Autodesk Inventor part; units mm, degrees
ref_plane "YZ Plane" through (0, 0, 0) normal (1, 0, 0) x (0, 1, 0)
ref_plane "XZ Plane" through (0, 0, 0) normal (0, 1, 0) x (-1, 0, 0)
ref_plane "XY Plane" through (0, 0, 0) normal (0, 0, 1) x (1, 0, 0)
sketch "Sketch1" plane through (0, 0, 0) normal (1, 0, 0) x (0, 1, 0)
  line L0 (0, 0) -> (12.4509, 21.5656)
  line L1 (12.4509, 21.5656) -> (46.5463, 1.8806)
  line L2 (0, -101.8491) -> (0, 42.1347)
  line L3 (46.5463, 1.8806) -> (0, -78.74)
  line L4 (0, 0) -> (0, -78.74)
  line L5 (19.05, 17.7556) -> (0, -15.24) construction
  dimension "d0" = 39.37
  dimension "d1" = 30
  dimension "d5" = 7.62
  dimension "d6" = 38.1
extrude "Extrusion1" add sketch "Sketch1" along normal mid plane 39.37
sketch "Sketch2" plane through (-19.685, 12.4509, 21.5656) normal (0, 0.5, 0.866) x (1, 0, 0)
  line L0 (0, 0) -> (39.37, 0) construction
  line L1 (39.37, 0) -> (39.37, 39.37) construction
  line L2 (0, 0) -> (39.37, 39.37) construction
  line L3 (39.37, 39.37) -> (0, 39.37) construction
  line L4 (0, 39.37) -> (39.37, 0) construction
  line L5 (6.35, 6.35) -> (33.02, 6.35)
  line L6 (33.02, 6.35) -> (33.02, 33.02)
  line L7 (33.02, 33.02) -> (6.35, 33.02)
  line L8 (6.35, 33.02) -> (6.35, 6.35)
  line L9 (6.35, 6.35) -> (33.02, 33.02) construction
  line L10 (33.02, 6.35) -> (6.35, 33.02) construction
  point P0 (19.685, 0)
  point P1 (19.685, 19.685)
  dimension "d7" = 26.67
extrude "Extrusion2" cut sketch "Sketch2" against normal blind 38.1
sketch "Sketch3" plane through (0, 0, 0) normal (1, 0, 0) x (0, 1, 0)
  line L0 (12.4509, 21.5656) -> (0, 0)
  line L1 (0, 0) -> (0, -78.74)
  line L2 (0, -78.74) -> (46.5463, 1.8806)
  line L3 (21.997, -27.94) -> (0, -15.24)
  line L4 (17.9501, 18.3906) -> (0, -12.7)
  line L5 (0, 0) -> (0, -78.74)
  line L6 (12.4509, 21.5656) -> (-1.0999, 21.5656) construction
  line L7 (0, 0) -> (12.4509, 21.5656)
  line L8 (0, 0) -> (0, 59.6656)
  line L9 (46.5463, 1.8806) -> (0, -78.74)
  line L10 (0, -78.74) -> (0, -104.14)
  line L11 (0, -137.4091) -> (0, 77.6947)
  line L12 (0, 59.6656) -> (-9.525, 59.6656)
  line L13 (-9.525, 59.6656) -> (-9.525, -104.14)
  line L14 (-9.525, -104.14) -> (0, -104.14)
  point P0 (1.0999, -13.335)
  point P1 (0, -15.24)
  point P2 (0, -12.7)
  dimension "d10" = 38.1
  dimension "d11" = 25.4
  dimension "d12" = 9.525
  dimension "supportBaseLength" = 163.8056
extrude "Extrusion3" add sketch "Sketch3" along normal mid plane 25.4
sketch "Sketch5" plane through (0, 0, 0) normal (1, 0, 0) x (0, 1, 0)
  line L0 (0, 0) -> (12.4509, 21.5656)
  line L1 (0, 59.6656) -> (0, 0)
  line L2 (12.4509, 21.5656) -> (46.5463, 1.8806)
  line L3 (12.4509, 21.5656) -> (0, 21.5656)
  line L4 (0, 0) -> (12.4509, 21.5656)
extrude "Extrusion5" add sketch "Sketch5" along normal mid plane 25.4
sketch "Sketch4" plane through (0, 0, 0) normal (0, 0, 1) x (1, 0, 0)
  line L0 (19.685, 46.5463) -> (-19.685, 46.5463)
  line L1 (19.685, 0) -> (19.685, 46.5463)
  line L2 (19.685, 0) -> (12.7, 0)
  line L3 (12.7, 0) -> (-12.7, 0)
  line L4 (-12.7, 0) -> (-19.685, 0)
  line L5 (-19.685, 46.5463) -> (-19.685, 0)
  line L6 (-12.7, 0) -> (-12.7, -9.525)
  line L7 (12.7, -9.525) -> (-12.7, -9.525)
  line L8 (12.7, -9.525) -> (12.7, 0)
  line L9 (-12.7, 0) -> (-19.685, 6.985)
  line L10 (-19.685, 46.5463) -> (-19.685, 0)
  line L11 (-19.685, 6.985) -> (-19.685, 0)
  line L12 (0, 0) -> (0, 46.5463) construction
  line L13 (12.7, 0) -> (19.685, 0)
  line L14 (12.7, 0) -> (19.685, 6.985)
  line L15 (19.685, 6.985) -> (19.685, 0)
  dimension "d15" = 45
extrude "Extrusion4" cut sketch "Sketch4" against normal up to surface (163.8056 mm away) from surface at 59.6656 contours L1 L2 L14 | L9 L4 L5
sketch "Sketch6" plane through (-12.7, 0, 59.6656) normal (0, 1, 0) x (1, 0, 0)
  line L0 (25.4, 163.8056) -> (0, 163.8056) construction
  line L1 (12.7, 163.8056) -> (12.7, 0) construction
  line L2 (25.4, 0) -> (0, 0) construction
  point P0 (12.7, 59.6656)
  point P1 (12.7, 151.1056)
  point P2 (12.7, 12.7)
  dimension "d21" = 12.7
  dimension "d22" = 12.7
hole "Hole1" at (0, 0, -91.44) at (0, 0, 46.9656) direction (0, -1, 0) diameter 5.6134 end through all
sketch "Sketch9" plane through (0, 0, 0) normal (1, 0, 0) x (0, 1, 0)
  line L0 (0.635, -11.6001) -> (0.635, -15.6066)
  line L1 (0.635, -15.6066) -> (21.997, -27.94)
  line L2 (41.047, 5.0556) -> (21.997, -27.94)
  line L3 (17.9501, 18.3906) -> (41.047, 5.0556)
  line L4 (17.9501, 18.3906) -> (0.635, -11.6001)
  line L5 (29.4986, 11.7231) -> (10.4486, -21.2725) construction
  line L6 (0.635, -15.6066) -> (21.997, -27.94) construction
  circle A0 centre (19.9736, -4.7747) radius 2.8067
  point P0 (0, 0)
  dimension "d30" = 5.6134
extrude "Extrusion6" cut sketch "Sketch9" along normal through all both and the other way through all contours A0
sketch "Sketch10" plane through (-19.685, 46.5463, 1.8806) normal (0, 0.866, -0.5) x (1, 0, 0)
  line L0 (6.35, 0) -> (33.02, 0) construction
  line L1 (19.685, 0) -> (19.685, 77.7875) construction
  point P0 (19.685, 24.9018)
  point P1 (19.685, 19.05)
  dimension "d33" = 19.05
hole "Hole2" at (0, 37.0213, -14.6172) direction (0, -0.866, 0.5) diameter 5.6134 depth 6.35
equation "\"d0\" = widthToSupportExtrusion"
equation "\"d1\" = attachementAngle"
equation "\"d6\" = insertDepth"
equation "\"d2\" = widthToSupportExtrusion"
equation "\"d7\" = insertForExtrusion"
equation "\"d8\" = insertDepth"
equation "\"d10\" = lenghtUnderBrace"
equation "\"d11\" = backLength"
equation "\"d12\" = supportBaseDepth"
equation "\"d13\" = supportBaseWidth"
equation "\"d19\" = supportBaseWidth"
equation "\"attachementAngle\" = 30deg"
equation "\"extrusionSize\" = 25.4"
equation "\"wallThickness\" = 6.35"
equation "\"slipClearance\" = 0.635"
equation "\"insertForExtrusion\" = extrusionSize + 2 * slipClearance"
equation "\"widthToSupportExtrusion\" = insertForExtrusion + 2 * wallThickness"
equation "\"insertDepth\" = 38.1"
equation "\"supportBaseWidth\" = 25.4"
equation "\"supportBaseDepth\" = 9.525"
equation "\"supportHoleDistanceFromEnd\" = 12.7"
equation "\"lenghtUnderBrace\" = 38.1"
equation "\"backLength\" = 25.4"
properties part number "30DegreeAttachementV03"
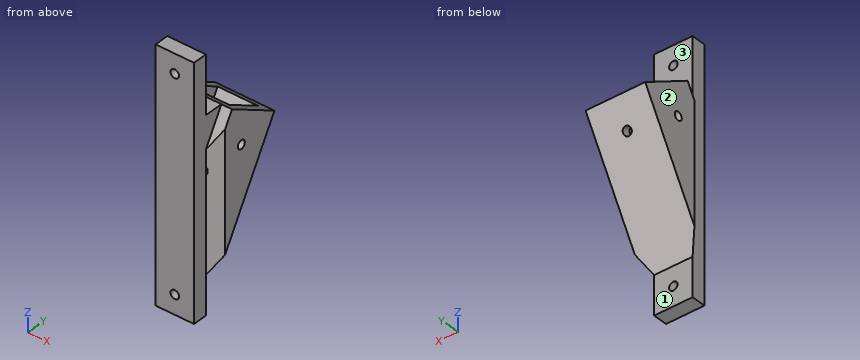
The model under review builds one solid part; all positions refer to its coordinate system, in mm. Face numbers are marked on the shaded views. A direction names the side the tool comes from. Give positions to 0.01 mm unless a question says otherwise; leave off trailing zeros. Order: outer loops, then holes, each group sorted by start corner. A loop starts at its lowest first (then second) coordinate and runs counter-clockwise, first axis right, second up. Notation, with made-up numbers: M -31,89.25 L -1,89.25 A17 cw -1,114.25 Z; hole C 71,13 d7. An arc over 180 degrees is marked long. Use one line per item in the form item = value. Start each with the question number.
Item 1: For the marked faces 1, 2 and 3, list the 3-axis set-ups (+Z, -Z, +X, -X, +Y, -Y) from which the entire face can be reached by the end or side of a thin tool; tool diameter is ignored.
Item 2: Insertion check: pin 1 Ø12.5 at (x, z) = (1, -86.5) entering from +Y; pin 2 Ø6 at (x, y) = (-0.5, 4.5) entering from +Z; pin 3 Ø6.5 at (y, z) = (2.5, -15.5) entering from +X. Each pin has a flat end and moves straight along its axis. Give the tip position at first contact, or say it passes through.
Item 3: We need section C-C on x = 7.5. Give the boundary of the cut face in (y, z) (3 decimals), plus the area to 3 significant figures.
Item 4: We need section B-B on x = 0. Give the boundary of the cut face in (y, z) (3 decimals), plus the area to 3 significant figures.
Item 5: We need section D-D on z = -43. Give the boundary of the cut face in (x, y) (3 decimals), plus the area to 3 significant figures.
Item 6: To check wall thickness, follow line 1 along Z through (x, y) = (0, -3); line 2 along X through (y, z) = (-3, -91); line 3 along X through (y, z) = (10, -2) (3 decimals). State the ranges of each line that lie inside material, in increasing order. Write a range as from..to.
Item 7: We need section A-A on z = -91.44. Give the boundary of the cut face in (x, y) (3 decimals), plus the area to 3 significant figures.
Completed:
q1.face_1 = -Z, +X, -X, +Y
q1.face_2 = +Z, -Z, -X, +Y, -Y
q1.face_3 = +Z, +X, -X, +Y
q2.pin_1 = 0
q2.pin_2 = 21.57
q2.pin_3 = 18.45
q3.outline = M -9.525,-104.14 L 0,-104.14 L 0,-78.74 L 46.546,1.881 L 41.047,5.056 L 21.996,-27.942 L 0,-15.242 L 0,-12.7 L 17.95,18.391 L 12.451,21.566 L 0,21.566 L 0,59.666 L -9.525,59.666 Z
q3.area = 3,000 mm²
q4.outline = M -9.525,-104.14 L 0,-104.14 L 0,-94.247 L -9.525,-94.247 Z; M -9.525,-88.633 L 0,-88.633 L 0,-78.74 L 35.618,-17.048 L 30.119,-13.873 L 21.996,-27.942 L 0,-15.242 L 0,-12.7 L 17.95,18.391 L 12.451,21.566 L 0,21.566 L 0,44.159 L -9.525,44.159 Z; M -9.525,49.772 L 0,49.772 L 0,59.666 L -9.525,59.666 Z; M 32.925,-9.012 L 38.425,-12.187 L 46.546,1.881 L 41.047,5.056 Z
q4.area = 2,860 mm²
q5.outline = M -19.685,6.985 L -12.7,0 L -12.7,-9.525 L 12.7,-9.525 L 12.7,0 L 19.685,6.985 L 19.685,20.634 L -19.685,20.634 Z
q5.area = 1,010 mm²
q6.line_1 = -104.14..-94.25, -88.63..44.16, 49.77..59.67
q6.line_2 = -12.7..-2.77, 2.77..12.7
q6.line_3 = -19.685..-13.335, 13.335..19.685
q7.outline = M -12.7,-9.525 L -2.807,-9.525 L -2.807,0 L -12.7,0 Z; M 2.807,-9.525 L 12.7,-9.525 L 12.7,0 L 2.807,0 Z
q7.area = 188 mm²
